The listing builds one solid part. Answer for the finished solid, in the listing's coordinates (mm). A direction names the side the tool comes from. Coordinates: 2 decimals unless noted, no trailing zeros. Write each loop counter-clockwise with the first axis right and the second up, starting at its lowest first coordinate (ties: lowest second). Pieces come first, ordered by that corner, then holes.
(1) The part is cut by section B-B on x = -14. Determine the outline of the cut face in (y, z), plus the area to 3 significant figures.
(2) Which of the six approach directions +Z, -Z, +X, -X, +Y, -Y give full straight-line access (tool end or side, diameter ignored) to faces 1 (the cylindrical face through (-0.391, -28.776, 48.986)), 2 (the flat face through (-26, 33.15, 41)), 3 (the flat face through (-23.798, -31, 41)), 4 (the flat face through (0, 26.1, 48))?
(3) The part is cut by section A-A on y = 15. Determine the outline of the cut face in (x, z), plus the area to 3 significant figures.
(4) The part is cut by section D-D on x = 24.5. Determine the outline of the cut face in (y, z), plus the area to 3 significant figures.
(5) Straight lines are drawn through the part: line 1 (Y direction, x = -6, z = 46.5); line 2 (Y direction, x = -14, z = 47.65); line 3 (Y direction, x = -27, z = 42.5). For each, find the intervals that lie inside material, in ascending order.
(6) For a pull along Y with two mould halves and no side action, classify faces 5 (the cylindrical face through (-14.202, 32.037, 47.972)), 6 (the flat face through (-29, 0, 47.9)), 7 (the cylindrical face through (-14.34, 34.58, 49.4)), 8 (the flat face through (-26, -33.15, 41)) as +Y half, -Y half, draft (parallel to the pull), parting line (faces both ways), or undercut.
(7) Given P1, Ø8, axis at x = -6.5, z = 40, coming from the -Y side; P2, Ø1.1, axis at y = -12.5, z = 48.5, coming from the -X side; P3, Ø1.4, axis at y = -30.5, z = 41, coming from the +X side; P4, Ø1.6, axis at x = 31, y = 14, coming from the -Z side, each flat-ended and moving along its own axis, determine where each tip first touches the part or whether it passes through.
(8) The part is cut by section C-C on z = 43. Determine the outline of the cut face in (x, y).
from build123d import *

# Parameters (mm, degrees)
SKETCH077_W          = 62
SKETCH077_H          = 70.3
SKETCH077_R          = 1.75
SKETCH077_R_2        = 1.55
SKETCH077_W_2        = 52.2
SKETCH077_H_2        = 52.2
PAD021_DEPTH         = 4
FILLET009_R          = 2
SKETCH078_W          = 2
SKETCH078_H          = 2.1
POCKET050_DEPTH      = 35.151
POCKET050_DEPTH_BACK = 35.151
SKETCH079_R          = 3
POCKET028_DEPTH      = 2.001
SKETCH081_W          = 4.202
SKETCH081_H          = 4.8
PAD023_DEPTH         = 10
CHAMFER003_SIZE2     = 9.99
CHAMFER003_SIZE      = 1.99


with BuildPart() as part:
    # Sketch077 → Pad021 (new body)
    with BuildSketch(Plane.XY):
        with Locations((1, 0)):
            Rectangle(SKETCH077_W, SKETCH077_H)
        with Locations((0, 31.75)):
            Circle(SKETCH077_R, mode=Mode.SUBTRACT)
        with Locations((0, -31.75)):
            Circle(SKETCH077_R, mode=Mode.SUBTRACT)
        with Locations((-14, 30.5)):
            Circle(SKETCH077_R_2, mode=Mode.SUBTRACT)
        Rectangle(SKETCH077_W_2, SKETCH077_H_2, mode=Mode.SUBTRACT)
    extrude(amount=PAD021_DEPTH)

    # Fillet009
    fillet009_edges = [part.edges().sort_by_distance(p)[0] for p in [
        (1, 35.15, 4),
        (1, -35.15, 4),
    ]]
    fillet(fillet009_edges, radius=FILLET009_R)

    # Sketch078 → Pocket050 (cut, two sides)
    with BuildSketch(Plane.XZ) as pocket050_sk:
        with Locations((-29, 2.95)):
            Rectangle(SKETCH078_W, SKETCH078_H)
        with Locations((31, 1.05)):
            Rectangle(SKETCH078_W, SKETCH078_H)
    extrude(amount=-POCKET050_DEPTH, mode=Mode.SUBTRACT)
    extrude(pocket050_sk.sketch, amount=POCKET050_DEPTH_BACK, mode=Mode.SUBTRACT)

    # Sketch079 → Pocket028 (cut, through all)
    with BuildSketch(Plane.XY.offset(2)):
        with Locations((0, -31.75)):
            Circle(SKETCH079_R)
        with Locations((0, 31.75)):
            Circle(SKETCH079_R)
    extrude(amount=POCKET028_DEPTH, mode=Mode.SUBTRACT)

    # Sketch081 → Pad023 (join)
    with BuildSketch(Plane.XY):
        with Locations((-25.899, 30.75)):
            Rectangle(SKETCH081_W, SKETCH081_H)
        with Locations((-25.899, -30.75)):
            Rectangle(SKETCH081_W, SKETCH081_H)
    extrude(amount=-PAD023_DEPTH)

    # Chamfer003
    chamfer003_edges = [part.edges().sort_by_distance(p)[0] for p in [
        (-28, 30.75, 0),
        (-28, -30.75, 0),
    ]]
    chamfer003_side = part.faces().sort_by_distance((-29.075766, 0, 0))[0]
    chamfer(chamfer003_edges, length=CHAMFER003_SIZE, length2=CHAMFER003_SIZE2, reference=chamfer003_side)


with BuildPart() as part_1:
    # Body058 placement: moved
    add(part.part.moved(Location((0, 0, 46))))


solid = part_1.part
Model answer:
1. outline: (-35.15, 46) - (-26.1, 46) - (-26.1, 50) - (-33.15, 50) arc R2 ccw to (-35.15, 48) - close; (26.1, 46) - (28.95, 46) - (28.95, 50) - (26.1, 50) - close; (32.05, 46) - (35.15, 46) - (35.15, 48) arc R2 ccw to (33.15, 50) - (32.05, 50) - close
1. area: 58.3 mm2
2. face 1: +Z
2. face 2: -Z, +X, -X, +Y
2. face 3: -Z, +X, +Y, -Y
2. face 4: +Z, -Z
3. outline: (-30, 46) - (-26.1, 46) - (-26.1, 50) - (-28, 50) - (-28, 47.9) - (-30, 47.9) - close; (26.1, 46) - (30, 46) - (30, 48.1) - (32, 48.1) - (32, 50) - (26.1, 50) - close
3. area: 30.8 mm2
4. outline: (-35.15, 46) - (-26.1, 46) - (-26.1, 50) - (-33.15, 50) arc R2 ccw to (-35.15, 48) - close; (26.1, 46) - (35.15, 46) - (35.15, 48) arc R2 ccw to (33.15, 50) - (26.1, 50) - close
4. area: 70.7 mm2
5. line 1: y = -35.15 to -26.1, 26.1 to 35.15
5. line 2: y = -35.15 to -26.1, 26.1 to 28.95, 32.05 to 35.15
5. line 3: y = -33.15 to -28.35, 28.35 to 33.15
6. face 5: undercut
6. face 6: draft
6. face 7: +Y half
6. face 8: -Y half
7. P1: passes through
7. P2: stops at x = -28
7. P3: stops at x = -23.8
7. P4: stops at z = 48.1
8. outline: (-29.39, -33.15) - (-23.8, -33.15) - (-23.8, -28.35) - (-29.39, -28.35) - close; (-29.39, 28.35) - (-23.8, 28.35) - (-23.8, 33.15) - (-29.39, 33.15) - close
